```python
from build123d import *

# Parameters (mm, degrees)
CYLINDER_R     = 4.76
CYLINDER_DEPTH = 15
BOX_W          = 15
BOX_H          = 15
BOX_DEPTH      = 10


with BuildPart() as cylinder:
    # Cylinder → Cylinder (new body)
    with BuildSketch(Plane(origin=(7, 7, -3), x_dir=(1, 0, 0), z_dir=(0, 0, 1))):
        Circle(CYLINDER_R)
    extrude(amount=CYLINDER_DEPTH)


with BuildPart() as cut:
    # Box → Box (new body)
    with BuildSketch(Plane.XY):
        with Locations((7.5, 7.5)):
            Rectangle(BOX_W, BOX_H)
    extrude(amount=BOX_DEPTH)

    # Cut: cut Cylinder
    add(cylinder.part, mode=Mode.SUBTRACT)


solid = cut.part
```
Design review of the part built by this model. Coordinates are the model's own, in mm. Coordinates: 2 decimals unless noted, no trailing zeros. Write each loop counter-clockwise with the first axis right and the second up, starting at its lowest first coordinate (ties: lowest second). Pieces come first, ordered by that corner, then holes.
1) Add section A-A (y = 7). Write out the cut boundary in (x, z).
2) Add section C-C (z = 1.5). Write out the cut boundary in (x, y).
3) To check wall thickness, follow L1, parallel to X at y = 7, z = 4.5; L2, parallel to X at y = 5.5, z = 7. State the ranges of each line that lie inside material, in increasing order.
4) Insertion check: pin 1 (4 mm diameter, centred on x = 12.5, y = 5, fed in from -Z); pin 2 (8.5 mm diameter, centred on x = 7, y = 7, fed in from -Z). Each pin has a flat end and moves straight along its axis. Give the tip position at first contact, or say it passes through.
5) Mouldability with a two-part tool opening along Y and no side actions: class faces 1 (the flat face through (7, 0, 5)), 2 (the flat face through (7, 15, 5)), 3 (the cylindrical face through (11.54, 8.43, 4.93)), 4 (the flat face through (11, 11, 0)) as +Y half, -Y half, draft (parallel to the pull), parting line (faces both ways), or undercut.
Check result:
1. outline: (0, 0) - (2.24, 0) - (2.24, 10) - (0, 10) - close; (11.76, 0) - (15, 0) - (15, 10) - (11.76, 10) - close
2. outline: (0, 0) - (15, 0) - (15, 15) - (0, 15) - close; hole circle Ø9.52 at (7, 7)
3. L1: x = 0 to 2.24, 11.76 to 15
3. L2: x = 0 to 2.48, 11.52 to 15
4. pin 1: stops at z = 0
4. pin 2: passes through
5. face 1: -Y half
5. face 2: +Y half
5. face 3: undercut
5. face 4: draft
